```python
from build123d import *

# Parameters (mm, degrees)
SKETCH007_R  = 3
PAD003_DEPTH = 3
SKETCH008_R  = 1.5
PAD004_DEPTH = 7
FILLET_R     = 1
FILLET001_R  = 1


with BuildPart() as part:
    # Sketch007 → Pad003 (new body)
    with BuildSketch(Plane.XZ):
        with Locations((-30.848434, 32.311108)):
            Circle(SKETCH007_R)
    extrude(amount=PAD003_DEPTH)

    # Sketch008 → Pad004 (new body)
    with BuildSketch(Plane.XZ.offset(3)):
        with Locations((-30.848434, 32.311108)):
            Circle(SKETCH008_R)
    extrude(amount=PAD004_DEPTH)

    # Fillet
    fillet_edges = [part.edges().sort_by_distance(p)[0] for p in [
        (-32.348434, -3, 32.311108),
    ]]
    fillet(fillet_edges, radius=FILLET_R)

    # Fillet001
    fillet001_edges = [part.edges().sort_by_distance(p)[0] for p in [
        (-32.348434, -10, 32.311108),
    ]]
    fillet(fillet001_edges, radius=FILLET001_R)


solid = part.part
```
CAD build for the part. Positions are in the model's coordinates, mm. A direction names the side the tool comes from. Coordinates: 2 decimals unless noted, no trailing zeros. Order: outer loops, then holes, each group sorted by start corner. A loop starts at its lowest first (then second) coordinate and runs counter-clockwise, first axis right, second up.
(1) Drill centre lines: L1, parallel to Y at x = -31.2, z = 29.6; L2, parallel to X at y = -5.5, z = 32.35; L3, parallel to Y at x = -31.4, z = 30.5. Where is each one in solid material? Low to high.
Solution:
L1: y = -3 to 0
L2: x = -32.35 to -29.35
L3: y = -3.21 to 0
(2) Saw through at A-A, the plane y = -1. Write the cut outline in (x, z).
Solution:
outline: circle Ø6 at (-30.85, 32.31)
(3) Pin check, flat tips, straight feed: pin 1 Ø1.5 at (x, y) = (-30.5, -7.5) entering from -Z; pin 2 Ø1 at (y, z) = (-4.5, 33) entering from +X; pin 3 Ø2 at (y, z) = (-5.5, 34.5) entering from +X. Stop position of each tip, or through.
Solution:
pin 1: stops at z = 30.81
pin 2: stops at x = -29.36
pin 3: stops at x = -29.93
(4) Which spindle directions (+Z, -Z, +X, -X, +Y, -Y) get a long thin tool onto all of the face, cutting with end or side? Do faces 1 (the face through (-31.499, -1.479, 29.382)), 2 (the face through (-33, -3, 34)). Say none if no direction does.
Solution:
face 1: +Y, -Y
face 2: -Y
(5) Saw through at B-B, the plane y = -8.5. Write the cut outline in (x, z).
Solution:
outline: circle Ø3 at (-30.85, 32.31)
